Can you work these out from the model? Positions are in its coordinate system, mm. A direction names the side the tool comes from. Round coordinates to 2 decimals unless told otherwise and drop trailing zeros. Order: outer loops, then holes, each group sorted by start corner. A loop starts at its lowest first (then second) coordinate and runs counter-clockwise, first axis right, second up. Notation, with made-up numbers: M 16,4.5 L 31,4.5 A28 ccw 31,24.5 Z; hole C 17,-32 d10. An arc over 180 degrees is marked long. One line per question, with ' | ' between items.
```python
from build123d import *

# Parameters (mm, degrees)
SKETCH_1_W          = 12
SKETCH_1_H          = 12
EXTRUDE_1_DEPTH     = 9.5
SKETCH_2_R          = 5.5
EXTRUDE_2_DEPTH     = 149.5
SKETCH_3_W          = 12
SKETCH_3_H          = 12
EXTRUDE_3_DEPTH     = 12.5
SKETCH_4_R          = 4
EXTRUDE_4_DEPTH     = 8
SKETCH_5_R          = 2
CUT_EXTRUDE_1_DEPTH = 178.5
CUT_EXTRUDE_START   = -6
SKETCH_6_R          = 2.5
CUT_EXTRUDE_2_DEPTH = 6
FILLET_1_R          = 2


with BuildPart() as part:
    # 草图1 → 凸台-拉伸1 (new body)
    with BuildSketch(Plane.XY):
        Rectangle(SKETCH_1_W, SKETCH_1_H)
    extrude(amount=EXTRUDE_1_DEPTH)

    # 草图2 → 凸台-拉伸2 (add)
    with BuildSketch(Plane.XY.offset(9.5)):
        Circle(SKETCH_2_R)
    extrude(amount=EXTRUDE_2_DEPTH)

    # 草图3 → 凸台-拉伸3 (add)
    with BuildSketch(Plane.XY.offset(159)):
        Rectangle(SKETCH_3_W, SKETCH_3_H)
    extrude(amount=EXTRUDE_3_DEPTH)

    # 草图4 → 凸台-拉伸4 (add)
    with BuildSketch(Plane.XY.offset(171.5)):
        Circle(SKETCH_4_R)
    extrude(amount=EXTRUDE_4_DEPTH)

    # 草图5 → 切除-拉伸1 (cut)
    with BuildSketch(Plane.XY.offset(179.5)):
        Circle(SKETCH_5_R)
    extrude(amount=-CUT_EXTRUDE_1_DEPTH, mode=Mode.SUBTRACT)

    # 草图6 → 切除-拉伸2 (cut)
    with BuildSketch(Plane(origin=(0, 6, 0), x_dir=(1, 0, 0), z_dir=(0, 1, 0)).offset(CUT_EXTRUDE_START)):
        with Locations((0, -4.75)):
            Circle(SKETCH_6_R)
        with Locations((0, -163.75)):
            Circle(SKETCH_6_R)
    extrude(amount=CUT_EXTRUDE_2_DEPTH, mode=Mode.SUBTRACT)

    # 圆角1
    fillet_1_edges = [part.edges().sort_by_distance(p)[0] for p in [
        (6, -6, 165.25),
        (6, 6, 165.25),
        (-6, 6, 165.25),
        (-6, -6, 165.25),
        (6, -6, 4.75),
        (-6, -6, 4.75),
        (-6, 6, 4.75),
        (6, 6, 4.75),
    ]]
    fillet(fillet_1_edges, radius=FILLET_1_R)


solid = part.part
```
(1) Thinking about a two-plate mould opening in Z: for faces 4 (the flat face through (0, 6, 167)), 5 (the flat face through (-2, -1, 179.5)), 6 (the cylindrical face through (-2.498, 3.625, 4.64)), which applies, released by +Z, released by -Z, zero draft, split by the parting line, or undercut?
Final values:
face 4: zero draft | face 5: released by +Z | face 6: undercut
(2) If we section it at B-B on z = 38: Please give me the cut outline in (x, y), plus the area to 3 significant figures.
Final values:
outline: C 0,0 d11; hole C 0,0 d4 | area: 82.5 mm^2
(3) If we section it at C-C on z = 4.75: Please give me the cut outline in (x, y).
Final values:
outline: M -6,-4 A2 ccw -4,-6 L 4,-6 A2 ccw 6,-4 L 6,4 A2 ccw 4,6 L 2.5,6 L 2.5,0 L 2,0 A2 cw -2,0 L -2.5,0 L -2.5,6 L -4,6 A2 ccw -6,4 Z
(4) Please list where these lines run through material, in increasing order: probe 1 along Z at (x, y) = (0, 4.75); probe 2 along X at (y, z) = (2.5, 163.75); probe 3 along Z at (x, y) = (0, 2.25). Write a range as [from, to].
Final values:
probe 1: [0, 2.25], [7.25, 161.25], [166.25, 171.5] | probe 2: [-6, -2.5], [2.5, 6] | probe 3: [0, 2.25], [7.25, 161.25], [166.25, 179.5]
(5) If we section it at A-A on x = 0: Please give me the cut outline in (y, z), plus the area to 3 significant figures.
Final values:
outline: M -6,0 L 6,0 L 6,2.25 L 2,2.25 L 2,1 L -2,1 L -2,179.5 L -4,179.5 L -4,171.5 L -6,171.5 L -6,159 L -5.5,159 L -5.5,9.5 L -6,9.5 Z; M 2,7.25 L 6,7.25 L 6,9.5 L 5.5,9.5 L 5.5,159 L 6,159 L 6,161.25 L 2,161.25 Z; M 2,166.25 L 6,166.25 L 6,171.5 L 4,171.5 L 4,179.5 L 2,179.5 Z | area: 1,220 mm^2
(6) Will these pins go through, and if not, where does the flat tip stop? pin 1 Ø1.5 at (x, z) = (2, 52) entering from +Y; pin 2 Ø6 at (y, z) = (4.5, 114.5) entering from +X; pin 3 Ø4 at (x, z) = (-2, 80.5) entering from -Y.
Final values:
pin 1: y = 5.36 | pin 2: x = 5.29 | pin 3: y = -5.5
(7) On a 3-axis mill with a long thin cutter (end or side, diameter ignored), from which of +Z, -Z, +X, -X, +Y, -Y can I reach the whole of each face in a straight line? I mean faces 1 (the cylindrical face through (-2.498, 3.625, 163.64)), 2 (the cylindrical face through (-1.19, -5.37, 83.2)), 3 (the cylindrical face through (0, -2, 91)). Say none if no direction works.
Final values:
face 1: +Y | face 2: none | face 3: +Z
